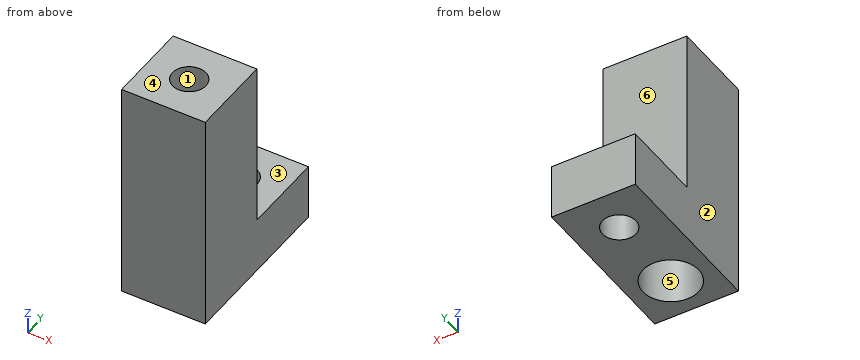
from build123d import *

# Parameters (mm, degrees)
F0_W     = 15
F0_H     = 15
F0_R     = 3
F1_DEPTH = 40
F2_W     = 15
F2_H     = 15
F2_R     = 3
F3_DEPTH = 10
F4_R     = 5
F5_DEPTH = 25


with BuildPart() as f1:
    # F0 (on Top) → F1 (new body)
    with BuildSketch(Plane.XY):
        Rectangle(F0_W, F0_H)
        Circle(F0_R, mode=Mode.SUBTRACT)
    extrude(amount=F1_DEPTH)

    # F2 (on face) → F3 (join)
    with BuildSketch(Plane(origin=(0, 0, 0), x_dir=(1, 0, 0), z_dir=(0, 0, -1))):
        with Locations((0, -15)):
            Rectangle(F2_W, F2_H)
        with Locations((0, -15)):
            Circle(F2_R, mode=Mode.SUBTRACT)
    extrude(amount=-F3_DEPTH)

    # F4 (on face) → F5 (cut)
    with BuildSketch(Plane(origin=(0, 0, 0), x_dir=(1, 0, 0), z_dir=(0, 0, -1))):
        Circle(F4_R)
    extrude(amount=-F5_DEPTH, mode=Mode.SUBTRACT)


solid = f1.part
Geometry check sheet. Reference: the model listing, model coordinates, mm. Face numbers are marked on the shaded views. A direction names the side the tool comes from. Give positions to 0.01 mm unless a question says otherwise; leave off trailing zeros. Loops run counter-clockwise (first coordinate to the right, second up) from the corner with the lowest first, then second, coordinate; pieces in that order, holes last. Notation, with made-up numbers: (-3, 0) -> (52, 0) arc R18 ccw to (52, 35) -> close; hole circle Ø5 at (72, 11.5). An arc over 180 degrees is marked (long way). Answer in a Markdown table with one row per item. Add a question column.
1) Gauge pin test, flat ends, axial feed: P1, Ø3, axis at x = 2, y = -1, coming from the -Z side; P2, Ø6, axis at x = 0.5, y = 17, coming from the +Z side; P3, Ø3.5, axis at x = 0, y = 0, coming from the -Z side; P4, Ø8, axis at x = 0, y = 0, coming from the +Z side. Record the tip position at first contact, or that the pin passes through.
2) Material ranges on probe 1 along Y at (x, z) = (0, 6.5); probe 2 along Y at (x, z) = (0, 30.25); probe 3 along Y at (x, z) = (0, 11.5), recorded low to high. Write a range as from..to.
3) Set-up check for the marked faces 4, 5 and 6: record each of +Z, -Z, +X, -X, +Y, -Y from which the full face is reachable in a straight line by a thin tool's end or side.
4) Cross-section at D-D on z = 9. Record the boundary of the cut face in (x, y).
5) Cross-section at B-B on y = 15. Record the boundary of the cut face in (x, z).
6) Draft check along X on the marked faces 1, 2 and 3. Enter one of: pulls with the +X half, pulls with the -X half, needs draft (parallel to the pull), parting line crosses it, or undercut.
7) Cross-section at A-A on x = 0. Record the boundary of the cut face in (y, z).
8) Cross-section at C-C on x = -4. Record the boundary of the cut face in (y, z).
Outcome:
| question | item | result |
|---|---|---|
| 1 | P1 | stops at z = 25 |
| 1 | P2 | stops at z = 10 |
| 1 | P3 | passes through |
| 1 | P4 | stops at z = 40 |
| 2 | probe 1 | y = -7.5..-5, 5..12, 18..22.5 |
| 2 | probe 2 | y = -7.5..-3, 3..7.5 |
| 2 | probe 3 | y = -7.5..-5, 5..7.5 |
| 3 | face 4 | +Z, +X, -X, +Y, -Y |
| 3 | face 5 | -Z |
| 3 | face 6 | +Z, +X, -X, +Y |
| 4 | outline | (-7.5, -7.5) -> (7.5, -7.5) -> (7.5, 22.5) -> (-7.5, 22.5) -> close; hole circle Ø10 at (0, 0); hole circle Ø6 at (0, 15) |
| 5 | outline | (-7.5, 0) -> (-3, 0) -> (-3, 10) -> (-7.5, 10) -> close; (3, 0) -> (7.5, 0) -> (7.5, 10) -> (3, 10) -> close |
| 6 | face 1 | undercut |
| 6 | face 2 | pulls with the -X half |
| 6 | face 3 | needs draft |
| 7 | outline | (-7.5, 0) -> (-5, 0) -> (-5, 25) -> (-3, 25) -> (-3, 40) -> (-7.5, 40) -> close; (3, 25) -> (5, 25) -> (5, 0) -> (12, 0) -> (12, 10) -> (7.5, 10) -> (7.5, 40) -> (3, 40) -> close; (18, 0) -> (22.5, 0) -> (22.5, 10) -> (18, 10) -> close |
| 8 | outline | (-7.5, 0) -> (-3, 0) -> (-3, 25) -> (3, 25) -> (3, 0) -> (22.5, 0) -> (22.5, 10) -> (7.5, 10) -> (7.5, 40) -> (-7.5, 40) -> close |
